```python
from build123d import *

# Parameters (mm, degrees)
EXTRUDE_1_DEPTH     = 3
SKETCH_3_R          = 8.5
EXTRUDE_2_DEPTH     = 4
FILLET_1_R          = 2
SKETCH_4_R          = 6.5
CUT_EXTRUDE_1_DEPTH = 1
SKETCH_5_R          = 6.5
EXTRUDE_3_DEPTH     = 10
CHAMFER_1_SIZE      = 1
SKETCH_6_R          = 4.5
CUT_EXTRUDE_2_DEPTH = 15


with BuildPart() as part:
    # Эскиз1 → Бобышка-Вытянуть1 (new body)
    with BuildSketch(Plane(origin=(0, 0, 0), x_dir=(1, 0, 0), z_dir=(0, 1, 0))):
        Polygon((9.814954576, 0), (4.907477288, 8.5), (-4.907477288, 8.5), (-9.814954576, 0), (-4.907477288, -8.5), (4.907477288, -8.5), align=None)
    extrude(amount=EXTRUDE_1_DEPTH)

    # Эскиз2 → Вырез-Повернуть2 (revolve, cut)
    with BuildSketch(Plane.XY):
        Polygon((9.814954576, 1), (8.814954576, 0), (9.814954576, 0), align=None)
    cut_revolve_2 = revolve(axis=Axis((0, 10.488289755, 0), (0, -1, 0)), mode=Mode.SUBTRACT)

    # Зеркальное отражение1: Вырез-Повернуть2 across plane
    add(cut_revolve_2.mirror(Plane.ZX.offset(1.5)), mode=Mode.SUBTRACT)

    # Эскиз3 → Бобышка-Вытянуть2 (add)
    with BuildSketch(Plane(origin=(0, 3, 0), x_dir=(1, 0, 0), z_dir=(0, 1, 0))):
        with Locations(Location((0, 0, 0), (0, 0, 270))):
            Circle(SKETCH_3_R)
    extrude(amount=EXTRUDE_2_DEPTH)

    # Скругление1
    fillet_1_edges = [part.edges().sort_by_distance(p)[0] for p in [
        (0, 7, -8.5),
    ]]
    fillet(fillet_1_edges, radius=FILLET_1_R)

    # Эскиз4 → Вырез-Вытянуть1 (cut)
    with BuildSketch(Plane(origin=(0, 7, 0), x_dir=(1, 0, 0), z_dir=(0, 1, 0))):
        with Locations(Location((0, 0, 0), (0, 0, 270))):
            Circle(SKETCH_4_R)
    extrude(amount=-CUT_EXTRUDE_1_DEPTH, mode=Mode.SUBTRACT)

    # Эскиз5 → Бобышка-Вытянуть3 (add)
    with BuildSketch(Plane.XZ):
        with Locations(Location((0, 0, 0), (0, 0, 90))):
            Circle(SKETCH_5_R)
    extrude(amount=EXTRUDE_3_DEPTH)

    # Фаска1
    chamfer_1_edges = [part.edges().sort_by_distance(p)[0] for p in [
        (0, -10, -6.5),
    ]]
    chamfer(chamfer_1_edges, length=CHAMFER_1_SIZE)

    # Эскиз6 → Вырез-Вытянуть2 (cut)
    with BuildSketch(Plane.XZ.offset(10)):
        with Locations(Location((0, 0, 0), (0, 0, 270))):
            Circle(SKETCH_6_R)
    extrude(amount=-CUT_EXTRUDE_2_DEPTH, mode=Mode.SUBTRACT)


solid = part.part
```
Source: CAD feature listing. Evaluate the final solid. Frame: model axes, mm. A direction names the side the tool comes from. Coordinates: 2 decimals unless noted, no trailing zeros. Write each loop counter-clockwise with the first axis right and the second up, starting at its lowest first coordinate (ties: lowest second). Pieces come first, ordered by that corner, then holes. Notation, with made-up numbers: (-7.5, 32) -> (25.5, 32) arc R18 cw to (25.5, 64) -> close; hole circle Ø3 at (69.5, -16). An arc over 180 degrees is marked (long way). Return JSON: item names as keys, results as strings. Group by question number.
1) Mould query, pull axis Z, two halves, no side actions, for faces 4 (the face through (-3.955, 6.507, -5.158)), 5 (the face through (4.57, 2.73, 7.85)), 6 (the face through (4.515, 0.271, -7.885)). Classes: +Z half, -Z half, draft (parallel to the pull), parting line (faces both ways), or undercut.
2) Section query A-A, the plane y = 0.25. Return loops of the section in (x, z).
3) Section query B-B, the plane y = -4.5. Return loops of the section in (x, z).
4) Ray query, line 1 along X through (y, z) = (-4.5, 0); line 2 along Z through (x, y) = (-2, -4.25); line 3 along X through (y, z) = (6.75, 0). Return the intervals inside material, ascending.
5) Set-up query: faces 1 (the face through (4.8, 3, -7.2)), 2 (the face through (0, 5, 0)), 3 (the face through (0, 6, 0)). Return all of +Z, -Z, +X, -X, +Y, -Y with unobstructed straight access to the full face (end or side cutting, diameter ignored); none if empty.
6) Contact query for flat-ended pins moving along their axis: P1, Ø3, axis at x = 7, y = -7.5, coming from the -Z side; P2, Ø1.2, axis at x = -8, z = 1, coming from the +Y side; P3, Ø2, axis at x = -5.5, y = -3.5, coming from the +Z side. Output: stop coordinate, or through.
From the geometry:
{
 "1": {"face 4": "undercut", "face 5": "+Z half", "face 6": "-Z half"},
 "2": {"outline": "(-8.94, -1.52) -> (-5.79, -6.98) arc R9.06 ccw to (-3.15, -8.5) -> (3.15, -8.5) arc R9.06 ccw to (5.79, -6.98) -> (8.94, -1.52) arc R9.06 ccw to (8.94, 1.52) -> (5.79, 6.98) arc R9.06 ccw to (3.15, 8.5) -> (-3.15, 8.5) arc R9.06 ccw to (-5.79, 6.98) -> (-8.94, 1.52) arc R9.06 ccw to start; hole circle Ø9 at (0, 0)"},
 "3": {"outline": "circle Ø13 at (0, 0); hole circle Ø9 at (0, 0)"},
 "4": {"line 1": "-6.5 to -4.5, 4.5 to 6.5", "line 2": "-6.18 to -4.03, 4.03 to 6.18", "line 3": "-7.47 to -6.5, 6.5 to 7.47"},
 "5": {"face 1": "-Z, +X, +Y", "face 2": "-Y", "face 3": "+Y"},
 "6": {"P1": "z = -3.46", "P2": "y = 6.75", "P3": "z = 4.69"}
}
